The model under review builds one solid part; all positions refer to its coordinate system, in mm. Coordinates: 2 decimals unless noted, no trailing zeros. Write each loop counter-clockwise with the first axis right and the second up, starting at its lowest first coordinate (ties: lowest second). Pieces come first, ordered by that corner, then holes.
1) For line 1 (X direction, y = 0.9, z = -364.5); line 2 (X direction, y = 2.2, z = -202.5); line 3 (Y direction, x = 4.75, z = -366), list the stretches that pass through material, from the lowest coordinate up.
2) For P1, Ø1.2, axis at x = 2.5, z = -35, coming from the +Y side; P2, Ø1.8, axis at x = 3, z = -79.5, coming from the +Y side, all flat-tipped, find the tip position at first contact; note any pin that passes through.
3) Add section B-B, the plane z = -251.5. State the section outline as (x, y) points, then the cut area to 3 significant figures.
4) Add section A-A, the plane y = 0.6. Give the number of separate pieces and of enclosed holes in the cut face, then the cut area to 3 significant figures.
from build123d import *

# Parameters (mm, degrees)
SKETCH1_W           = 5
SKETCH1_H           = 3.7
BOSS_EXTRUDE1_DEPTH = 400
SKETCH2_R           = 1.75
CUT_EXTRUDE1_DEPTH  = 2
SKETCH3_R           = 1
CUT_EXTRUDE2_DEPTH  = 401.036248358
CUT_EXTRUDE3_DEPTH  = 401.048359577


with BuildPart() as part:
    # Sketch1 → Boss-Extrude1 (new body)
    with BuildSketch(Plane.XY):
        with Locations((2.5, 1.85)):
            Rectangle(SKETCH1_W, SKETCH1_H)
    extrude(amount=-BOSS_EXTRUDE1_DEPTH)

    # Sketch2 → Cut-Extrude1 (cut)
    with BuildSketch(Plane(origin=(0, 3.7, 0), x_dir=(1, 0, 0), z_dir=(0, 1, 0))):
        with Locations(Location((2.5, 5, 0), (0, 0, 270))):
            Circle(SKETCH2_R)
        with Locations(Location((2.5, 20, 0), (0, 0, 270))):
            Circle(SKETCH2_R)
        with Locations(Location((2.5, 35, 0), (0, 0, 270))):
            Circle(SKETCH2_R)
        with Locations(Location((2.5, 50, 0), (0, 0, 270))):
            Circle(SKETCH2_R)
        with Locations(Location((2.5, 65, 0), (0, 0, 270))):
            Circle(SKETCH2_R)
        with Locations(Location((2.5, 80, 0), (0, 0, 270))):
            Circle(SKETCH2_R)
        with Locations(Location((2.5, 95, 0), (0, 0, 270))):
            Circle(SKETCH2_R)
        with Locations(Location((2.5, 110, 0), (0, 0, 270))):
            Circle(SKETCH2_R)
        with Locations(Location((2.5, 125, 0), (0, 0, 270))):
            Circle(SKETCH2_R)
        with Locations(Location((2.5, 140, 0), (0, 0, 270))):
            Circle(SKETCH2_R)
        with Locations(Location((2.5, 155, 0), (0, 0, 270))):
            Circle(SKETCH2_R)
        with Locations(Location((2.5, 170, 0), (0, 0, 270))):
            Circle(SKETCH2_R)
        with Locations(Location((2.5, 185, 0), (0, 0, 270))):
            Circle(SKETCH2_R)
        with Locations(Location((2.5, 200, 0), (0, 0, 270))):
            Circle(SKETCH2_R)
        with Locations(Location((2.5, 215, 0), (0, 0, 270))):
            Circle(SKETCH2_R)
        with Locations(Location((2.5, 230, 0), (0, 0, 270))):
            Circle(SKETCH2_R)
        with Locations(Location((2.5, 245, 0), (0, 0, 270))):
            Circle(SKETCH2_R)
        with Locations(Location((2.5, 260, 0), (0, 0, 270))):
            Circle(SKETCH2_R)
        with Locations(Location((2.5, 275, 0), (0, 0, 270))):
            Circle(SKETCH2_R)
        with Locations(Location((2.5, 290, 0), (0, 0, 270))):
            Circle(SKETCH2_R)
        with Locations(Location((2.5, 305, 0), (0, 0, 270))):
            Circle(SKETCH2_R)
        with Locations(Location((2.5, 320, 0), (0, 0, 270))):
            Circle(SKETCH2_R)
        with Locations(Location((2.5, 335, 0), (0, 0, 270))):
            Circle(SKETCH2_R)
        with Locations(Location((2.5, 350, 0), (0, 0, 270))):
            Circle(SKETCH2_R)
        with Locations(Location((2.5, 365, 0), (0, 0, 270))):
            Circle(SKETCH2_R)
        with Locations(Location((2.5, 380, 0), (0, 0, 270))):
            Circle(SKETCH2_R)
        with Locations(Location((2.5, 395, 0), (0, 0, 270))):
            Circle(SKETCH2_R)
    extrude(amount=-CUT_EXTRUDE1_DEPTH, mode=Mode.SUBTRACT)

    # Sketch3 → Cut-Extrude2 (cut, through all)
    with BuildSketch(Plane(origin=(0, 1.7, 0), x_dir=(1, 0, 0), z_dir=(0, 1, 0))):
        with Locations(Location((2.5, 5, 0), (0, 0, 270))):
            Circle(SKETCH3_R)
        with Locations(Location((2.5, 20, 0), (0, 0, 270))):
            Circle(SKETCH3_R)
        with Locations(Location((2.5, 35, 0), (0, 0, 270))):
            Circle(SKETCH3_R)
        with Locations(Location((2.5, 50, 0), (0, 0, 270))):
            Circle(SKETCH3_R)
        with Locations(Location((2.5, 65, 0), (0, 0, 270))):
            Circle(SKETCH3_R)
        with Locations(Location((2.5, 80, 0), (0, 0, 270))):
            Circle(SKETCH3_R)
        with Locations(Location((2.5, 95, 0), (0, 0, 270))):
            Circle(SKETCH3_R)
        with Locations(Location((2.5, 110, 0), (0, 0, 270))):
            Circle(SKETCH3_R)
        with Locations(Location((2.5, 125, 0), (0, 0, 270))):
            Circle(SKETCH3_R)
        with Locations(Location((2.5, 140, 0), (0, 0, 270))):
            Circle(SKETCH3_R)
        with Locations(Location((2.5, 155, 0), (0, 0, 270))):
            Circle(SKETCH3_R)
        with Locations(Location((2.5, 170, 0), (0, 0, 270))):
            Circle(SKETCH3_R)
        with Locations(Location((2.5, 185, 0), (0, 0, 270))):
            Circle(SKETCH3_R)
        with Locations(Location((2.5, 200, 0), (0, 0, 270))):
            Circle(SKETCH3_R)
        with Locations(Location((2.5, 215, 0), (0, 0, 270))):
            Circle(SKETCH3_R)
        with Locations(Location((2.5, 230, 0), (0, 0, 270))):
            Circle(SKETCH3_R)
        with Locations(Location((2.5, 245, 0), (0, 0, 270))):
            Circle(SKETCH3_R)
        with Locations(Location((2.5, 260, 0), (0, 0, 270))):
            Circle(SKETCH3_R)
        with Locations(Location((2.5, 275, 0), (0, 0, 270))):
            Circle(SKETCH3_R)
        with Locations(Location((2.5, 290, 0), (0, 0, 270))):
            Circle(SKETCH3_R)
        with Locations(Location((2.5, 305, 0), (0, 0, 270))):
            Circle(SKETCH3_R)
        with Locations(Location((2.5, 320, 0), (0, 0, 270))):
            Circle(SKETCH3_R)
        with Locations(Location((2.5, 335, 0), (0, 0, 270))):
            Circle(SKETCH3_R)
        with Locations(Location((2.5, 350, 0), (0, 0, 270))):
            Circle(SKETCH3_R)
        with Locations(Location((2.5, 365, 0), (0, 0, 270))):
            Circle(SKETCH3_R)
        with Locations(Location((2.5, 380, 0), (0, 0, 270))):
            Circle(SKETCH3_R)
        with Locations(Location((2.5, 395, 0), (0, 0, 270))):
            Circle(SKETCH3_R)
    extrude(amount=-CUT_EXTRUDE2_DEPTH, mode=Mode.SUBTRACT)

    # Sketch4 → Cut-Extrude3 (cut, through all)
    with BuildSketch(Plane.XY):
        Polygon((0, 2.7), (0.5, 2.2), (0, 1.7), align=None)
        Polygon((5, 2.7), (4.5, 2.2), (5, 1.7), align=None)
    extrude(amount=-CUT_EXTRUDE3_DEPTH, mode=Mode.SUBTRACT)


solid = part.part
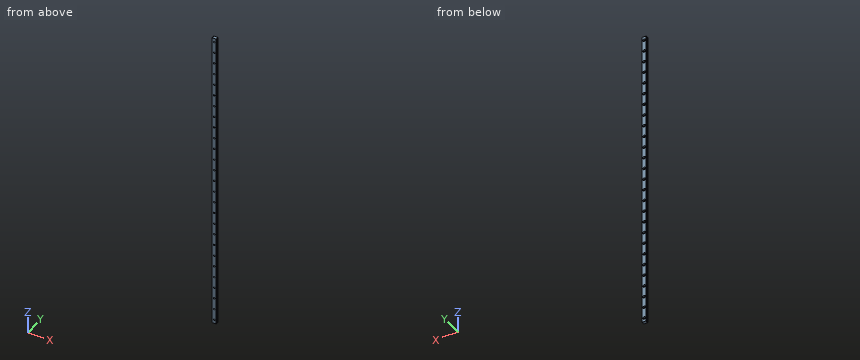
Geometry results:
1. line 1: x = 0 to 1.63, 3.37 to 5
1. line 2: x = 0.5 to 4.5
1. line 3: y = 0 to 1.95, 2.45 to 3.7
2. P1: passes through
2. P2: stops at y = 1.7
3. outline: (0, 0) - (5, 0) - (5, 1.7) - (4.5, 2.2) - (5, 2.7) - (5, 3.7) - (0, 3.7) - (0, 2.7) - (0.5, 2.2) - (0, 1.7) - close
3. area: 18.0 mm2
4. separate pieces: 1
4. enclosed holes: 27
4. area: 1,920 mm2
